The listing builds one solid part. Answer for the finished solid, in the listing's coordinates (mm). Face numbers are marked on the shaded views. A direction names the side the tool comes from. Coordinates: 2 decimals unless noted, no trailing zeros. Order: outer loops, then holes, each group sorted by start corner. A loop starts at its lowest first (then second) coordinate and runs counter-clockwise, first axis right, second up. Notation, with made-up numbers: M -33.5,85 L -28.5,85 A34 cw -28.5,117 Z; hole C -6.5,51.5 d4. An arc over 180 degrees is marked long. One line per item, written item: value. Start each with the question number.
Q1. For the marked faces 4, 5, 6 and 7, determine the directions among +Z, -Z, +X, -X, +Y, -Y from which every point of the face is accessible in a straight line to the end or side of a thin tool.
Q2. The part is cut by section A-A on z = 4. Give the vertices of the cut face in (x, y).
Q3. Straight lines are drawn through the part: line 1 along Z through (x, y) = (5, -0.2); line 2 along Y through (x, z) = (7, 6); line 3 along X through (y, z) = (-20.75, 5.25). For each, find the intervals that lie inside material, in ascending order. Write a range as [from, to].
Q4. Each of these flat-tipped pins is pushed along its axis until it touches: pin 1 Ø0.5 at (x, y) = (22.5, 0.5) entering from +Z; pin 2 Ø3 at (x, z) = (15.5, 8.5) entering from -Y; pin 3 Ø5 at (x, z) = (28.5, 6) entering from -Y. Where does it stop, or does it pass through?
Q5. The part is cut by section D-D on x = 17. Give the vertices of the cut face in (y, z).
Q6. The part is cut by section C-C on z = 2. Give the vertices of the cut face in (x, y).
Q7. The part is cut by section B-B on x = 5. Give the vertices of the cut face in (y, z).
Q8. Determine the mould class of the marked faces 1, 2 and 3 for opening direction X: pulls with the +X half, pulls with the -X half, needs draft (parallel to the pull), parting line crosses it, or undercut.
```python
from build123d import *

# Parameters (mm, degrees)
BOSS_EXTRU_1_DEPTH      = 10
ESQUISSE2_W             = 35
ESQUISSE2_H             = 2.9
BOSS_EXTRU_2_DEPTH      = 1
ESQUISSE3_W             = 35
ESQUISSE3_H             = 2.9
BOSS_EXTRU_3_DEPTH      = 1
ESQUISSE4_R             = 1.5
ENL_V_MAT_EXTRU_1_DEPTH = 5
ESQUISSE5_R             = 1.5
ENL_V_MAT_EXTRU_2_DEPTH = 22.5


with BuildPart() as part:
    # Esquisse1 → Boss.-Extru.1 (new body)
    with BuildSketch(Plane.XY):
        with BuildLine():
            Line((0, 0), (35, 0))
            Line((35, 0), (10.251262658, -24.748737342))
            Line((10.251262658, -24.748737342), (8.129942315, -22.627416998))
            Line((8.129942315, -22.627416998), (24.343145751, -6.414213562))
            ThreePointArc((24.343145751, -6.414213562), (24.776691253, -4.234633135), (22.928932188, -3))
            Line((22.928932188, -3), (0, -3))
            Line((0, -3), (0, 0))
        make_face()
    extrude(amount=BOSS_EXTRU_1_DEPTH)

    # Esquisse2 → Boss.-Extru.2 (add)
    with BuildSketch(Plane(origin=(0, 0, 0), x_dir=(1, 0, 0), z_dir=(0, 1, 0))):
        with Locations((17.5, -5)):
            Rectangle(ESQUISSE2_W, ESQUISSE2_H)
    extrude(amount=BOSS_EXTRU_2_DEPTH)

    # Esquisse3 → Boss.-Extru.3 (add)
    with BuildSketch(Plane(origin=(17.5, -17.5, 0), x_dir=(0.707106781, 0.707106781, 0), z_dir=(0.707106781, -0.707106781, 0))):
        with Locations((7.248737342, 5)):
            Rectangle(ESQUISSE3_W, ESQUISSE3_H)
    extrude(amount=BOSS_EXTRU_3_DEPTH)

    # Esquisse4 → Enlèv. mat.-Extru.1 (cut, through all)
    with BuildSketch(Plane.XZ.offset(3)):
        with Locations((5, 5)):
            Circle(ESQUISSE4_R)
        with Locations((15, 5)):
            Circle(ESQUISSE4_R)
    extrude(amount=-ENL_V_MAT_EXTRU_1_DEPTH, mode=Mode.SUBTRACT)

    # Esquisse5 → Enlèv. mat.-Extru.2 (cut, through all)
    with BuildSketch(Plane(origin=(15.378679656, -15.378679656, 0), x_dir=(0.707106781, 0.707106781, 0), z_dir=(-0.707106781, 0.707106781, 0))):
        with Locations((-5.251262658, -5)):
            Circle(ESQUISSE5_R)
        with Locations((4.748737342, -5)):
            Circle(ESQUISSE5_R)
    extrude(amount=-ENL_V_MAT_EXTRU_2_DEPTH, mode=Mode.SUBTRACT)


solid = part.part
```
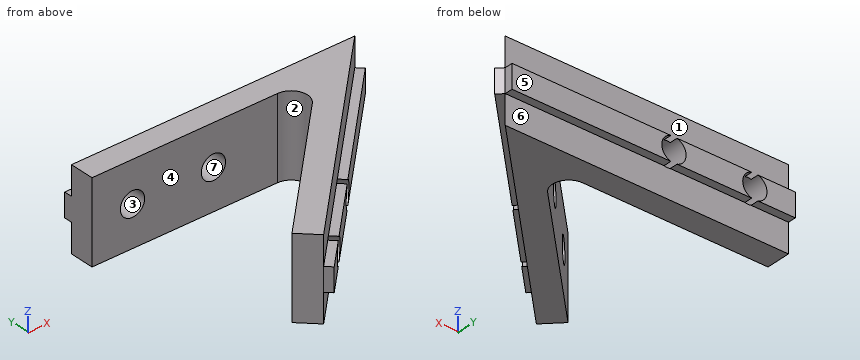
Output:
1. face 4: +Z, -Z, -X
1. face 5: +Z, -Z, +X, -X, +Y
1. face 6: -Z, +X, -X, +Y
1. face 7: +Y
2. outline: M 0,-3 L 3.88,-3 L 3.88,1 L 0,1 Z; M 6.12,-3 L 13.88,-3 L 13.88,1 L 6.12,1 Z; M 8.13,-22.63 L 10.96,-25.46 L 13.7,-22.71 L 10.87,-19.88 Z; M 12.46,-18.3 L 15.28,-21.13 L 20.77,-15.64 L 17.95,-12.81 Z; M 16.12,-3 L 22.93,-3 A2 cw 24.34,-6.41 L 19.53,-11.23 L 22.36,-14.06 L 35.71,-0.71 L 35,0 L 35,1 L 16.12,1 Z
3. line 1: z = [0, 3.5], [6.5, 10]
3. line 2: y = [-3, 1]
3. line 3: x = [10.01, 11.23], [15.42, 15.66]
4. pin 1: stops at z = 6.45
4. pin 2: stops at y = -21
4. pin 3: stops at y = -10.41
5. outline: M -19.41,3.55 L -18,3.55 L -18,0 L -13.76,0 L -13.76,10 L -18,10 L -18,6.45 L -19.41,6.45 Z; M -3,0 L 0,0 L 0,3.55 L 1,3.55 L 1,6.45 L 0,6.45 L 0,10 L -3,10 Z
6. outline: M 0,-3 L 22.93,-3 A2 cw 24.34,-6.41 L 8.13,-22.63 L 10.25,-24.75 L 35,0 L 0,0 Z
7. outline: M -3,0 L 0,0 L 0,3.5 L -3,3.5 Z; M -3,6.5 L 0,6.5 L 0,10 L -3,10 Z
8. face 1: needs draft
8. face 2: pulls with the -X half
8. face 3: undercut
